Design review of the part shown in the three views and the two pictorial views. Dimensions are in mm from the part's minimum x, y and z. A direction names the side the tool comes from. Give positions to 0.01 mm unless a question says otherwise; leave off trailing zeros. Order: outer loops, then holes, each group sorted by start corner. A loop starts at its lowest first (then second) coordinate and runs counter-clockwise, first axis right, second up. Notation, with made-up numbers: (9, 89) -> (42, 89) arc R8 cw to (42, 95) -> close; hole circle Ø1 at (57, 54.25). An arc over 180 degrees is marked (long way). Use one line per item in the form item = value.
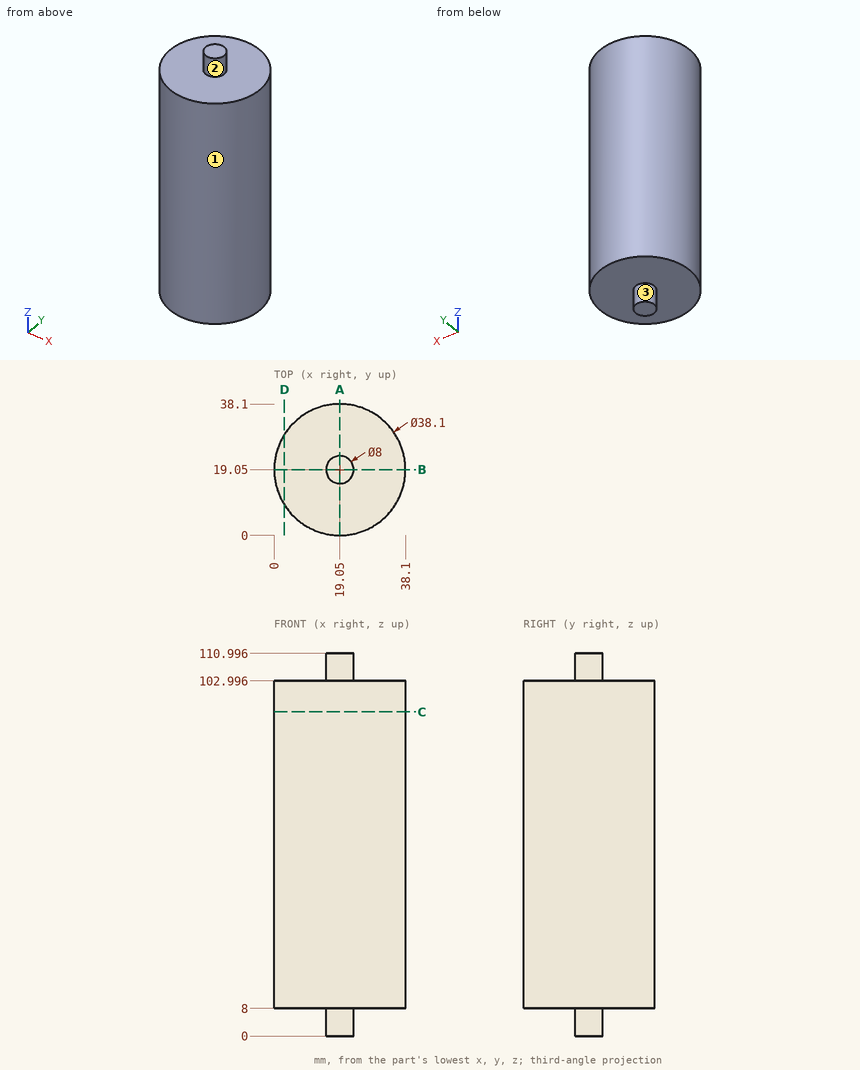
1. For pin 1 Ø1.5 at (y, z) = (25.5, 57.5) entering from +X; pin 2 Ø1.5 at (x, z) = (23.5, 22) entering from -Y; pin 3 Ø12 at (x, z) = (25, 91.5) entering from +Y, all flat-tipped, find the tip position at first contact; note any pin that passes through.
Values:
pin_1 = 37.23
pin_2 = 0.36
pin_3 = 38.1
2. Add section D-D on x = 3. Give the boundary of the cut face in (y, z), then the cut area to 3 significant figures.
Values:
outline = (8.79, 8) -> (29.31, 8) -> (29.31, 103) -> (8.79, 103) -> close
area = 1,950 mm^2
3. Add section A-A on x = 19.05. Give the boundary of the cut face in (y, z).
Values:
outline = (0, 8) -> (15.05, 8) -> (15.05, 0) -> (23.05, 0) -> (23.05, 8) -> (38.1, 8) -> (38.1, 103) -> (23.05, 103) -> (23.05, 111) -> (15.05, 111) -> (15.05, 103) -> (0, 103) -> close
4. Add section C-C on z = 94. Give the boundary of the cut face in (x, y).
Values:
outline = circle Ø38.1 at (19.05, 19.05)
5. Tool access review of the marked faces 1, 2 and 3: name each direction out of +Z, -Z, +X, -X, +Y, -Y from which nothing blocks a thin tool from reaching the whole face with its end or side.
Values:
face_1 = +Z, -Z
face_2 = +Z
face_3 = -Z
6. For L1, parallel to Z at x = 19, y = 11.5; L2, parallel to X at y = 24, z = 46; L3, parallel to X at y = 11, z = 95.5, list the stretches that pass through material, from the lowest coordinate up.
Values:
L1 = 8 to 103
L2 = 0.65 to 37.45
L3 = 1.78 to 36.32
